Could you check a few things on this model? Use its own coordinates, in mm. Round coordinates to 2 decimals unless told otherwise and drop trailing zeros. Loops run counter-clockwise (first coordinate to the right, second up) from the corner with the lowest first, then second, coordinate; pieces in that order, holes last. Notation, with made-up numbers: (83.5, 43.5) - (89.5, 43.5) arc R22 ccw to (89.5, 52.5) - close; hole circle Ø9 at (32, 6.25). An arc over 180 degrees is marked (long way). Use one line per item in the form item = value.
Autodesk Inventor part; units mm, degrees
ref_plane "YZ Plane" through (0, 0, 0) normal (1, 0, 0) x (0, 1, 0)
ref_plane "XZ Plane" through (0, 0, 0) normal (0, 1, 0) x (-1, 0, 0)
ref_plane "XY Plane" through (0, 0, 0) normal (0, 0, 1) x (1, 0, 0)
sketch "Sketch1" plane through (0, 0, 0) normal (1, 0, 0) x (0, 1, 0)
  circle A0 centre (0, 0) radius 19.5
  line L0 (43.5, 50) -> (-43.5, 50)
  line L1 (-43.5, 50) -> (-43.5, -50)
  line L2 (-43.5, -50) -> (43.5, -50)
  line L3 (43.5, -50) -> (43.5, 50)
  line L4 (43.5, 50) -> (-43.5, -50) construction
  line L5 (-43.5, 50) -> (43.5, -50) construction
  line L6 (0, 0) -> (0, -38)
  line L7 (0, -38) -> (34.15, -38)
  circle A1 centre (34.15, -38) radius 2.5
  circle A2 centre (-34.15, -38) radius 2.5
  circle A3 centre (34.15, 0) radius 2.5
  circle A4 centre (-34.15, 0) radius 2.5
  circle A5 centre (34.15, 38) radius 2.5
  circle A6 centre (-34.15, 38) radius 2.5
  dimension "d0" = 39
  dimension "d1" = 87
  dimension "d2" = 100
  dimension "d3" = 38
  dimension "d4" = 34.15
  dimension "d5" = 5
  dimension "d8" = 68.3
  dimension "d11" = 38
extrude "Extrusion1" add sketch "Sketch1" along normal blind 2
properties part number "mount_plate_4x2020" material "Aluminum 6061"
1. We'd pull the mould along Z, two halves only. Please class faces 1 (the face through (0.986, -2.539, -19.334)), 2 (the face through (1, -1, -50)), 3 (the face through (1, 1, 50)), 4 (the face through (1, 43.5, -1)): +Z half, -Z half, draft (parallel to the pull), parting line (faces both ways), or undercut.
Solution:
face_1 = undercut
face_2 = -Z half
face_3 = +Z half
face_4 = draft
2. Please list where these lines run through material, in increasing order: line 1 along Z through (x, y) = (1.2, 34.15); line 2 along Z through (x, y) = (1.2, 0); line 3 along Z through (x, y) = (1.8, 33.5).
Solution:
line_1 = -50 to -40.5, -35.5 to -2.5, 2.5 to 35.5, 40.5 to 50
line_2 = -50 to -19.5, 19.5 to 50
line_3 = -50 to -40.41, -35.59 to -2.41, 2.41 to 35.59, 40.41 to 50
3. If we section it at C-C, the plane y = -34.15: Write out the boundary of the cut face in (x, z).
Solution:
outline = (0, -50) - (2, -50) - (2, -40.5) - (0, -40.5) - close; (0, -35.5) - (2, -35.5) - (2, -2.5) - (0, -2.5) - close; (0, 2.5) - (2, 2.5) - (2, 35.5) - (0, 35.5) - close; (0, 40.5) - (2, 40.5) - (2, 50) - (0, 50) - close
4. For P1, Ø6.5, axis at y = 34.15, z = -38, coming from the -X side, with a flat end and sliding along its axis, tell me the tip position at first contact or that it passes through.
Solution:
P1 = 0
5. If we section it at D-D, the plane x = 1.5: Write out the boundary of the cut face in (y, z).
Solution:
outline = (-43.5, -50) - (43.5, -50) - (43.5, 50) - (-43.5, 50) - close; hole circle Ø5 at (-34.15, -38); hole circle Ø5 at (-34.15, 0); hole circle Ø5 at (-34.15, 38); hole circle Ø39 at (0, 0); hole circle Ø5 at (34.15, -38); hole circle Ø5 at (34.15, 0); hole circle Ø5 at (34.15, 38)
6. If we section it at B-B, the plane z = 0: Write out the boundary of the cut face in (x, y).
Solution:
outline = (0, -43.5) - (2, -43.5) - (2, -36.65) - (0, -36.65) - close; (0, -31.65) - (2, -31.65) - (2, -19.5) - (0, -19.5) - close; (0, 19.5) - (2, 19.5) - (2, 31.65) - (0, 31.65) - close; (0, 36.65) - (2, 36.65) - (2, 43.5) - (0, 43.5) - close
7. If we section it at A-A, the plane z = 38: Write out the boundary of the cut face in (x, y), plus the area to 3 significant figures.
Solution:
outline = (0, -43.5) - (2, -43.5) - (2, -36.65) - (0, -36.65) - close; (0, -31.65) - (2, -31.65) - (2, 31.65) - (0, 31.65) - close; (0, 36.65) - (2, 36.65) - (2, 43.5) - (0, 43.5) - close
area = 154 mm^2
